Could you check a few things on this drawing? It's one solid part, dimensions in mm from its lowest x, y, z. A direction names the side the tool comes from. Coordinates: 2 decimals unless noted, no trailing zeros. Write each loop counter-clockwise with the first axis right and the second up, starting at its lowest first coordinate (ties: lowest second). Pieces come first, ordered by that corner, then holes.
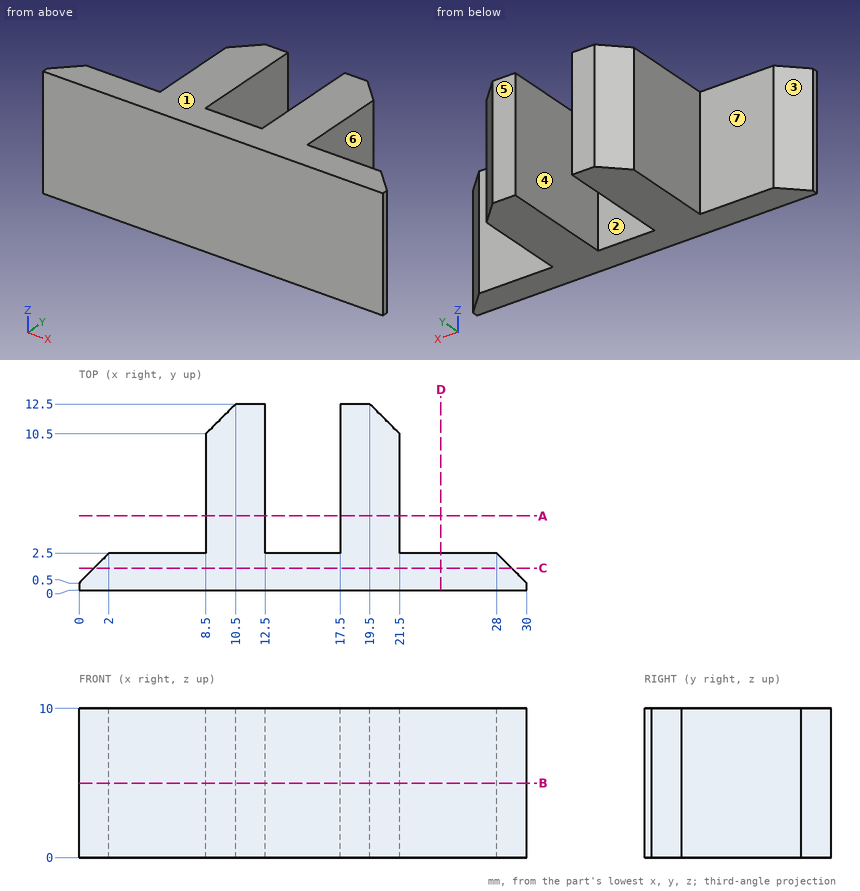
1) On a 3-axis mill with a long thin cutter (end or side, diameter ignored), from which of +Z, -Z, +X, -X, +Y, -Y can I reach the whole of each face in a straight line? I mean the marked faces 4, 5, 6 and 7. Say none if no direction works.
Values follow:
face 4: +Z, -Z, +Y
face 5: +Z, -Z, +X, -X, +Y
face 6: +Z, -Z, +X, +Y
face 7: +Z, -Z, -X, +Y
2) Imagine slicing it at A-A on y = 5. Please give me the cut outline in (x, z), then the cut area to 3 significant figures.
Values follow:
outline: (8.5, 0) - (12.5, 0) - (12.5, 10) - (8.5, 10) - close; (17.5, 0) - (21.5, 0) - (21.5, 10) - (17.5, 10) - close
area: 80.0 mm2
3) We'd pull the mould along X, two halves only. Please class the marked faces 1, 2 and 3: pulls with the +X half, pulls with the -X half, needs draft (parallel to the pull), parting line crosses it, or undercut.
Values follow:
face 1: needs draft
face 2: undercut
face 3: pulls with the -X half
4) Imagine slicing it at D-D on x = 24.25. Please give me the cut outline in (y, z).
Values follow:
outline: (0, 0) - (2.5, 0) - (2.5, 10) - (0, 10) - close
5) Imagine slicing it at C-C on y = 1.5. Please give me the cut outline in (x, z).
Values follow:
outline: (1, 0) - (29, 0) - (29, 10) - (1, 10) - close
6) Will these pins go through, and if not, where does the flat tip stop? pin 1 (2 mm diameter, centred on y = 8.5, z = 1.5, fed in from -X); pin 2 (2 mm diameter, centred on x = 26, z = 5.5, fed in from +Y); pin 3 (1.5 mm diameter, centred on x = 7.5, y = 10, fed in from -Z).
Values follow:
pin 1: stops at x = 8.5
pin 2: stops at y = 2.5
pin 3: passes through
7) I need wall thicknesses on probe 1 along X at (y, z) = (9.75, 8.5); probe 2 along Y at (x, z) = (26, 8.5); probe 3 along X at (y, z) = (10.75, 3.5). Which ranges of each line are inside material? Lowest first, please.
Values follow:
probe 1: x = 8.5 to 12.5, 17.5 to 21.5
probe 2: y = 0 to 2.5
probe 3: x = 8.75 to 12.5, 17.5 to 21.25
8) Imagine slicing it at B-B on z = 5. Please give me the cut outline in (x, y).
Values follow:
outline: (0, 0) - (30, 0) - (30, 0.5) - (28, 2.5) - (21.5, 2.5) - (21.5, 10.5) - (19.5, 12.5) - (17.5, 12.5) - (17.5, 2.5) - (12.5, 2.5) - (12.5, 12.5) - (10.5, 12.5) - (8.5, 10.5) - (8.5, 2.5) - (2, 2.5) - (0, 0.5) - close
